from build123d import *

# Parameters (mm, degrees)
EXTRUDE_THIN1_START             = 76.2
SKETCH5_W                       = 25.4
SKETCH5_H                       = 25.4
SKETCH5_W_2                     = 19.05
SKETCH5_H_2                     = 19.05
EXTRUDE_THIN1_DEPTH             = 736.6
F_5_0MM_DOWEL_HOLE1_D           = 5
F_5_0MM_DOWEL_HOLE1_CSINK_D     = 5.05
F_5_0MM_DOWEL_HOLE1_CSINK_ANGLE = 90


with BuildPart() as part:
    # Sketch5 → Extrude-Thin1 (new body)
    with BuildSketch(Plane(origin=(0, 0, 0), x_dir=(0, 0, -1), z_dir=(1, 0, 0)).offset(EXTRUDE_THIN1_START)):
        with Locations((101.6, 88.9)):
            Rectangle(SKETCH5_W, SKETCH5_H)
        with Locations((101.6, 88.9)):
            Rectangle(SKETCH5_W_2, SKETCH5_H_2, mode=Mode.SUBTRACT)
    extrude(amount=EXTRUDE_THIN1_DEPTH)

    # Ø5.0mm Dowel Hole1 (through all)
    with Locations(Plane(origin=(0, 76.2, 0), x_dir=(-1, 0, 0), z_dir=(0, -1, 0))):
        with Locations((-88.9, 107.95), (-88.9, 95.25), (-114.3, 107.95), (-114.3, 95.25), (-800.1, 107.95), (-800.1, 95.25)):
            CounterSinkHole(F_5_0MM_DOWEL_HOLE1_D / 2, F_5_0MM_DOWEL_HOLE1_CSINK_D / 2, counter_sink_angle=F_5_0MM_DOWEL_HOLE1_CSINK_ANGLE)


solid = part.part
Read the model definition and answer for the solid it produces. Units are mm, in the model's axes. A direction names the side the tool comes from. Give positions to 0.01 mm unless a question says otherwise; leave off trailing zeros. Write each loop counter-clockwise with the first axis right and the second up, starting at its lowest first coordinate (ties: lowest second). Pieces come first, ordered by that corner, then holes. Notation, with made-up numbers: (-13.5, 51) -> (36.5, 51) arc R29 ccw to (36.5, 89) -> close; hole circle Ø4 at (-26, 10.25). An arc over 180 degrees is marked (long way). Answer as a JSON object with one key per item and string values. Group by question number.
1) A tool of negligible diameter and unlimited length cuts with its end or side. For faces 1 (the flat face through (439, 89, -114.3)), 2 (the flat face through (439, 89, -92.075)), from which of +Z, -Z, +X, -X, +Y, -Y can it reach the whole face along a straight path? Write none if from no direction.
2) Consider L1, parallel to X at y = 77.2, z = -95.25; L2, parallel to Z at x = 88.9, y = 77.9; L3, parallel to Z at x = 772, y = 93 (3 decimals). Determine where each line is inside the solid, lowest interval first. Write a range as from..to.
3) Find section A-A (y = 86.75). Write down the section's boundary in (x, z) (3 decimals), and give its area (3 significant figures).
4) The mould has two halves that part along Y. Classify faces 3 (the flat face through (812.8, 89, -90)), 4 (the flat face through (439, 76.2, -101)), 5 (the flat face through (439, 101.6, -101)), 6 (the flat face through (439, 98.425, -101)): +Y half, -Y half, draft (parallel to the pull), parting line (faces both ways), or undercut.
5) Find section B-B (x = 418). Write down the section's boundary in (y, z) (3 decimals).
6) This flat-tipped pin is pushed along its axis until it touches: P1, Ø4, axis at x = 88.9, z = -107.95, coming from the +Y side. Where does it stop, or does it pass through?
Values follow:
{
 "1": {"face 1": "-Z, +X, -X, +Y, -Y", "face 2": "+X, -X"},
 "2": {"L1": "x = 76.2..86.4, 91.4..111.8, 116.8..797.6, 802.6..812.8", "L2": "z = -114.3..-110.45, -105.45..-97.75, -92.75..-88.9", "L3": "z = -114.3..-111.125, -92.075..-88.9"},
 "3": {"outline": "(76.2, -114.3) -> (812.8, -114.3) -> (812.8, -111.125) -> (76.2, -111.125) -> close; (76.2, -92.075) -> (812.8, -92.075) -> (812.8, -88.9) -> (76.2, -88.9) -> close", "area": "4,680 mm2"},
 "4": {"face 3": "draft", "face 4": "-Y half", "face 5": "+Y half", "face 6": "undercut"},
 "5": {"outline": "(76.2, -114.3) -> (101.6, -114.3) -> (101.6, -88.9) -> (76.2, -88.9) -> close; hole (79.375, -111.125) -> (98.425, -111.125) -> (98.425, -92.075) -> (79.375, -92.075) -> close"},
 "6": {"P1": "passes through"}
}
